```python
from build123d import *

# Parameters (mm, degrees)
F2_DEPTH       = 7.5
F3_R           = 13
F4_DEPTH       = 12
F5_R           = 5.5
F6_DEPTH       = 15.001
F7_R           = 7.49999
F9_D           = 5
F9_CBORE_D     = 10
F9_CBORE_DEPTH = 1
F11_DEPTH      = 2
F12_SIZE       = 1


# Not quite as in the source:
# - a fillet or chamfer is up to 0.001 mm smaller than in the source, because OpenCascade refuses the exact size


with BuildPart() as f2:
    # F1 (on Front) → F2 (new body, symmetric)
    with BuildSketch(Plane.XZ):
        with BuildLine():
            Line((-37.5, 0), (0, 0))
            Line((0, 0), (37.5, 0))
            Line((37.5, 0), (37.5, 4))
            Line((37.5, 4), (10.9544511501, 4))
            ThreePointArc((10.9544511501, 4), (9.0757782768, 5.3140056594), (9.6656921913, 7.5294117647))
            ThreePointArc((9.6656921913, 7.5294117647), (14.0900465494, 24.1449575543), (0, 34))
            ThreePointArc((0, 34), (-14.0900465494, 24.1449575543), (-9.6656921913, 7.5294117647))
            ThreePointArc((-9.6656921913, 7.5294117647), (-9.0757782768, 5.3140056594), (-10.9544511501, 4))
            Line((-10.9544511501, 4), (-37.5, 4))
            Line((-37.5, 4), (-37.5, 0))
        make_face()
    extrude(amount=F2_DEPTH, both=True)

    # F3 (on face) → F4 (cut)
    with BuildSketch(Plane.XZ.offset(7.5)):
        with Locations((0, 19)):
            Circle(F3_R)
    extrude(amount=-F4_DEPTH, mode=Mode.SUBTRACT)

    # F5 (on face) → F6 (cut, through all)
    with BuildSketch(Plane(origin=(0, 7.5, 0), x_dir=(-1, 0, 0), z_dir=(0, 1, 0))):
        with Locations((0, 19)):
            Circle(F5_R)
    extrude(amount=-F6_DEPTH, mode=Mode.SUBTRACT)

    # F7 (radius 7.5 in the source; OpenCascade refuses exactly that, so slightly less here)
    f7_edges = [f2.edges().sort_by_distance(p)[0] for p in [
        (37.5, -7.5, 2),
        (37.5, 7.5, 2),
        (-37.5, -7.5, 2),
        (-37.5, 7.5, 2),
    ]]
    fillet(f7_edges, radius=F7_R)

    # F9 (through all)
    with Locations(Plane.XY.offset(4)):
        with Locations((30, 0), (-30, 0)):
            CounterBoreHole(F9_D / 2, F9_CBORE_D / 2, F9_CBORE_DEPTH)

    # F10 (on Front) → F11 (join, symmetric)
    with BuildSketch(Plane.XZ):
        with BuildLine():
            Line((10.9544511501, 4), (24, 4))
            Line((24, 4), (13.4831460674, 25.5730337079))
            ThreePointArc((13.4831460674, 25.5730337079), (14.6751576274, 15.8952055444), (9.6656921913, 7.5294117647))
            ThreePointArc((9.6656921913, 7.5294117647), (9.0757782768, 5.3140056594), (10.9544511501, 4))
        make_face()
    extrude(amount=F11_DEPTH, both=True)

    # F12
    f12_edges = [f2.edges().sort_by_distance(p)[0] for p in [
        (5.5, 4.5, 19),
    ]]
    chamfer(f12_edges, length=F12_SIZE)

    # F13: F2 across plane


with BuildPart() as f2_1:
    add(f2.part)
    add(f2.part.mirror(Plane.YZ))


solid = f2_1.part
```
Source: CAD feature listing. Evaluate the final solid. Frame: model axes, mm. A direction names the side the tool comes from. Give positions to 0.01 mm unless a question says otherwise; leave off trailing zeros. Write each loop counter-clockwise with the first axis right and the second up, starting at its lowest first coordinate (ties: lowest second). Pieces come first, ordered by that corner, then holes.
1. First-contact query: pin 1 (6.5 mm diameter, centred on x = -30, y = 0, fed in from -Z); pin 2 (13 mm diameter, centred on x = 0, z = 20.5, fed in from -Y); pin 3 (5 mm diameter, centred on x = -31, y = -2, fed in from +Z); pin 4 (3 mm diameter, centred on y = 1, z = 23.5, fed in from -X) (3 decimals). Flat tips, straight axial feed; report the tip coordinate or a pass-through.
2. Access query for faces 5 (the face through (-18.815, -0.028, 14.636)), 6 (the face through (-6, 4.5, 16)), 7 (the face through (24.4, -0.1, 4)), 8 (the face through (-16, -2, 10)), 9 (the face through (-24, -3, 4)). Directions: +Z, -Z, +X, -X, +Y, -Y. A direction counts if a zero-diameter tool reaches every point of the face in a straight line with its end or side. Return the directions, or none.
3. Material intervals for line 1 along X through (y, z) = (0, 3.35); line 2 along X through (y, z) = (6.35, 19); line 3 along Y through (x, z) = (30, 3.55), sorted ascending.
4. Section query A-A (x = 0). Return the cut outline in (y, z), then the cut area to 3 significant figures.
5. Section query C-C (z = 19). Return the cut outline in (x, y), then the cut area to 4 significant figures.
6. Pull-direction query (X, two-part tool) for faces 1 (the face through (0.51, -0.11, 33.99)), 2 (the face through (-28, -2, 3)), 3 (the face through (-9.064, 4.712, 5.346)), 4 (the face through (16, -2, 10)); classes: +X half, -X half, draft (parallel to the pull), parting line (faces both ways), or undercut.
7. Section query B-B (y = -0.75). Return the cut outline in (x, z), then the cut area to 3 significant figures.
8. Section query D-D (y = -3.75). Return the cut outline in (x, z).
Output values:
1. pin 1: stops at z = 0
1. pin 2: stops at y = 4.5
1. pin 3: stops at z = 3
1. pin 4: stops at x = -15.225
2. face 5: +Z, -X, +Y, -Y
2. face 6: -Y
2. face 7: +X
2. face 8: -X, -Y
2. face 9: -X
3. line 1: x = -37.5 to -35, -25 to 25, 35 to 37.5
3. line 2: x = -15 to -5.5, 5.5 to 15
3. line 3: y = -7.5 to -5, 5 to 7.5
4. outline: (-7.5, 0) - (7.5, 0) - (7.5, 13.5) - (5.5, 13.5) - (4.5, 12.5) - (4.5, 6) - (-7.5, 6) - close; (-7.5, 32) - (4.5, 32) - (4.5, 25.5) - (5.5, 24.5) - (7.5, 24.5) - (7.5, 34) - (-7.5, 34) - close
4. area: 164 mm2
5. outline: (-16.69, -2) - (-15, -2) - (-15, -7.5) - (-13, -7.5) - (-13, 4.5) - (-6.5, 4.5) - (-5.5, 5.5) - (-5.5, 7.5) - (-15, 7.5) - (-15, 2) - (-16.69, 2) - close; (5.5, 5.5) - (6.5, 4.5) - (13, 4.5) - (13, -7.5) - (15, -7.5) - (15, -2) - (16.69, -2) - (16.69, 2) - (15, 2) - (15, 7.5) - (5.5, 7.5) - close
5. area: 117.5 mm2
6. face 1: parting line
6. face 2: undercut
6. face 3: -X half
6. face 4: draft
7. outline: (-37.46, 0) - (-32.38, 0) - (-32.38, 3) - (-34.94, 3) - (-34.94, 4) - (-37.46, 4) - close; (-27.62, 0) - (27.62, 0) - (27.62, 3) - (25.06, 3) - (25.06, 4) - (24, 4) - (13.48, 25.57) arc R15 ccw to (-13.48, 25.57) - (-24, 4) - (-25.06, 4) - (-25.06, 3) - (-27.62, 3) - close; (32.38, 0) - (37.46, 0) - (37.46, 4) - (34.94, 4) - (34.94, 3) - (32.38, 3) - close; hole circle Ø26 at (0, 19)
7. area: 692 mm2
8. outline: (-36.5, 0) - (36.5, 0) - (36.5, 4) - (33.31, 4) - (33.31, 3) - (26.69, 3) - (26.69, 4) - (10.95, 4) arc R2 cw to (9.67, 7.53) arc R15 ccw (long way) to (-9.67, 7.53) arc R2 cw to (-10.95, 4) - (-26.69, 4) - (-26.69, 3) - (-33.31, 3) - (-33.31, 4) - (-36.5, 4) - close; hole circle Ø26 at (0, 19)
